from build123d import *

# Parameters (mm, degrees)
BOSS_EXTRUDE1_DEPTH     = 11
CUT_EXTRUDE1_DEPTH      = 20.874606914
CUT_EXTRUDE1_DEPTH_BACK = 20.874606914
SKETCH3_W               = 11.85
SKETCH3_H               = 1.196323822
BOSS_EXTRUDE2_DEPTH     = 11
CHAMFER1_SIZE           = 1
FILLET1_R               = 1
SKETCH4_R               = 1.175
CUT_EXTRUDE2_DEPTH      = 21.326822777
CUT_EXTRUDE3_START      = 3
SKETCH5_R               = 2.25
SKETCH5_R_2             = 1.939534676
CUT_EXTRUDE3_DEPTH      = 10
FILLET2_R               = 2
FILLET3_R               = 1
CHAMFER2_SIZE           = 1


# Some blends are built 0.0001 mm under size
with BuildPart() as part:
    # Sketch1 → Boss-Extrude1 (new body)
    with BuildSketch(Plane.XY):
        with BuildLine():
            Line((-3.15, 0), (-15, 0))
            Line((-15, 0), (-15, 7))
            Line((-15, 7), (15, 7))
            Line((15, 7), (15, 0))
            Line((15, 0), (3.15, 0))
            ThreePointArc((3.15, 0), (0, 3.15), (-3.15, 0))
        make_face()
    extrude(amount=BOSS_EXTRUDE1_DEPTH)

    # Sketch2 → Cut-Extrude1 (cut, two sides: drawn at the far end of the back side and taken through both)
    with BuildSketch(Plane.XY.offset(11).offset(-CUT_EXTRUDE1_DEPTH_BACK)):
        Polygon((-9, 5.75), (0, 7), (-15, 7), (-15, 2.504439372), align=None)
        Polygon((15, 7), (0, 7), (9, 5.75), (15, 2.504439372), align=None)
    extrude(amount=CUT_EXTRUDE1_DEPTH + CUT_EXTRUDE1_DEPTH_BACK, mode=Mode.SUBTRACT)

    # Sketch3 → Boss-Extrude2 (add)
    with BuildSketch(Plane.XY.offset(11)):
        with Locations((-9.075, -0.598161911)):
            Rectangle(SKETCH3_W, SKETCH3_H)
        with Locations((9.075, -0.598161911)):
            Rectangle(SKETCH3_W, SKETCH3_H)
    extrude(amount=-BOSS_EXTRUDE2_DEPTH)

    # Chamfer1
    chamfer1_edges = [part.edges().sort_by_distance(p)[0] for p in [
        (15, 0.654057775, 11),
        (-15, 0.654057775, 0),
        (-15, 0.654057775, 11),
        (15, 0.654057775, 0),
    ]]
    chamfer(chamfer1_edges, length=CHAMFER1_SIZE)

    # Fillet1
    fillet1_edges = [part.edges().sort_by_distance(p)[0] for p in [
        (-3.15, -1.196323822, 5.5),
        (3.15, -1.196323822, 5.5),
    ]]
    fillet(fillet1_edges, radius=FILLET1_R)

    # Sketch4 → Cut-Extrude2 (cut, through all)
    with BuildSketch(Plane.XZ.offset(1.196323822)):
        with Locations(Location((-5.25, 3.5, 0), (0, 0, 20.581969212))):
            Circle(SKETCH4_R)
        with Locations((5.25, 3.5)):
            Circle(SKETCH4_R)
        with Locations((-11, 4)):
            Circle(SKETCH4_R)
        with Locations((11, 4)):
            Circle(SKETCH4_R)
    extrude(amount=-CUT_EXTRUDE2_DEPTH, mode=Mode.SUBTRACT)

    # Sketch5 → Cut-Extrude3 (cut)
    with BuildSketch(Plane(origin=(0, 0, 0), x_dir=(1, 0, 0), z_dir=(0, 1, 0)).offset(CUT_EXTRUDE3_START)):
        with Locations(Location((-5.25, -3.5, 0), (0, 0, 180))):
            Circle(SKETCH5_R)
        with Locations((5.25, -3.5)):
            Circle(SKETCH5_R)
        with Locations(Location((-11, -4, 0), (0, 0, 27.266044451))):
            Circle(SKETCH5_R)
        with Locations((11, -4)):
            Circle(SKETCH5_R_2)
    extrude(amount=CUT_EXTRUDE3_DEPTH, mode=Mode.SUBTRACT)

    # Fillet2
    # the kernel refuses this fillet: 2 mm, written as the material it takes off along each edge
    with BuildSketch(Plane(origin=(9, 5.75, -2.170275709), x_dir=(-0.9904922731777516, 0.13756837127468827, 0), z_dir=(0, 0, 1))) as fillet2_piece_1:
        with BuildLine():
            CenterArc((FILLET2_R * 0.180856309082, FILLET2_R), FILLET2_R, 249.497020474, 20.502979526)
            Line((-FILLET2_R * 0.169399781042, FILLET2_R * 0.0633460236933), (-FILLET2_R * 0.176404902844, FILLET2_R * 0.0446129441672))
            Line((-FILLET2_R * 0.176404902844, FILLET2_R * 0.0446129441672), (-FILLET2_R * 0.00361712618164, -FILLET2_R * 0.02))
            Line((-FILLET2_R * 0.00361712618164, -FILLET2_R * 0.02), (FILLET2_R * 0.180856309082, -FILLET2_R * 0.02))
            Line((FILLET2_R * 0.180856309082, -FILLET2_R * 0.02), (FILLET2_R * 0.180856309082, 0))
        make_face()
    extrude(amount=15.340551418, mode=Mode.SUBTRACT)
    with BuildSketch(Plane(origin=(-9, 5.75, 5.139499303), x_dir=(-0.879564366325619, -0.4757799128696085, 0), z_dir=(0, 0, -1))) as fillet2_piece_2:
        with BuildLine():
            CenterArc((FILLET2_R * 0.180856309082, -FILLET2_R), FILLET2_R, 90, 20.502979526)
            Line((-FILLET2_R * 0.169399781042, -FILLET2_R * 0.0633460236933), (-FILLET2_R * 0.176404902844, -FILLET2_R * 0.0446129441672))
            Line((-FILLET2_R * 0.176404902844, -FILLET2_R * 0.0446129441672), (-FILLET2_R * 0.00361712618164, FILLET2_R * 0.02))
            Line((-FILLET2_R * 0.00361712618164, FILLET2_R * 0.02), (FILLET2_R * 0.180856309082, FILLET2_R * 0.02))
            Line((FILLET2_R * 0.180856309082, FILLET2_R * 0.02), (FILLET2_R * 0.180856309082, 0))
        make_face()
    extrude(amount=7.309775012, mode=Mode.SUBTRACT)
    with BuildSketch(Plane(origin=(-9, 5.75, 13.170275709), x_dir=(-0.879564366325619, -0.4757799128696085, 0), z_dir=(0, 0, -1))) as fillet2_piece_3:
        with BuildLine():
            CenterArc((FILLET2_R * 0.180856309082, -FILLET2_R), FILLET2_R, 90, 20.502979526)
            Line((-FILLET2_R * 0.169399781042, -FILLET2_R * 0.0633460236933), (-FILLET2_R * 0.176404902844, -FILLET2_R * 0.0446129441672))
            Line((-FILLET2_R * 0.176404902844, -FILLET2_R * 0.0446129441672), (-FILLET2_R * 0.00361712618164, FILLET2_R * 0.02))
            Line((-FILLET2_R * 0.00361712618164, FILLET2_R * 0.02), (FILLET2_R * 0.180856309082, FILLET2_R * 0.02))
            Line((FILLET2_R * 0.180856309082, FILLET2_R * 0.02), (FILLET2_R * 0.180856309082, 0))
        make_face()
    extrude(amount=10.309775012, mode=Mode.SUBTRACT)
    with BuildSketch(Plane(origin=(0, 7, 12.666666667), x_dir=(-0.9904922731777517, -0.13756837127468774, 0), z_dir=(0, 0, -1))) as fillet2_piece_4:
        with BuildLine():
            CenterArc((FILLET2_R * 0.138888888889, -FILLET2_R), FILLET2_R, 90, 15.814325406)
            Line((-FILLET2_R * 0.133631928674, -FILLET2_R * 0.0378501135503), (-FILLET2_R * 0.139082345025, -FILLET2_R * 0.0186071158213))
            Line((-FILLET2_R * 0.139082345025, -FILLET2_R * 0.0186071158213), (-FILLET2_R * 0.00277777777778, FILLET2_R * 0.02))
            Line((-FILLET2_R * 0.00277777777778, FILLET2_R * 0.02), (FILLET2_R * 0.138888888889, FILLET2_R * 0.02))
            Line((FILLET2_R * 0.138888888889, FILLET2_R * 0.02), (FILLET2_R * 0.138888888889, 0))
        make_face()
    extrude(amount=14.333333333, mode=Mode.SUBTRACT)
    with BuildSketch(Plane(origin=(-15, 2.504439372, -6.151996245), x_dir=(0.8795643663256194, 0.4757799128696078, 0), z_dir=(0, 0, 1))) as fillet2_piece_5:
        with BuildLine():
            CenterArc((FILLET2_R * 0.595999687118, -FILLET2_R), FILLET2_R, 90, 61.589857771)
            Line((-FILLET2_R * 0.283564679207, -FILLET2_R * 0.52422008713), (-FILLET2_R * 0.301155966534, -FILLET2_R * 0.514704488873))
            Line((-FILLET2_R * 0.301155966534, -FILLET2_R * 0.514704488873), (-FILLET2_R * 0.0119199937424, FILLET2_R * 0.02))
            Line((-FILLET2_R * 0.0119199937424, FILLET2_R * 0.02), (FILLET2_R * 0.595999687118, FILLET2_R * 0.02))
            Line((FILLET2_R * 0.595999687118, FILLET2_R * 0.02), (FILLET2_R * 0.595999687118, 0))
        make_face()
    extrude(amount=23.303992491, mode=Mode.SUBTRACT)
    with BuildSketch(Plane(origin=(15, 2.504439372, -6.151996245), x_dir=(-0.87956436632562, 0.47577991286960686, 0), z_dir=(0, 0, 1))) as fillet2_piece_6:
        with BuildLine():
            CenterArc((FILLET2_R * 0.595999687118, FILLET2_R), FILLET2_R, 208.410142229, 61.589857771)
            Line((-FILLET2_R * 0.283564679207, FILLET2_R * 0.52422008713), (-FILLET2_R * 0.301155966534, FILLET2_R * 0.514704488873))
            Line((-FILLET2_R * 0.301155966534, FILLET2_R * 0.514704488873), (-FILLET2_R * 0.0119199937424, -FILLET2_R * 0.02))
            Line((-FILLET2_R * 0.0119199937424, -FILLET2_R * 0.02), (FILLET2_R * 0.595999687118, -FILLET2_R * 0.02))
            Line((FILLET2_R * 0.595999687118, -FILLET2_R * 0.02), (FILLET2_R * 0.595999687118, 0))
        make_face()
    extrude(amount=23.303992491, mode=Mode.SUBTRACT)

    # Fillet3
    fillet3_edges = [part.edges().sort_by_distance(p)[0] for p in [
        (15, -1.196323822, 5.5),
        (-15, -1.196323822, 5.5),
    ]]
    fillet(fillet3_edges, radius=FILLET3_R)

    # Chamfer2
    chamfer2_edges = [part.edges().sort_by_distance(p)[0] for p in [
        (-11.634854678, 4.324736566, 0),
        (-11.634854678, 4.324736566, 11),
        (-8.989888283, 5.719170071, 0),
        (-8.989888283, 5.719170071, 11),
        (-4.458431595, 6.38077339, 0),
        (-4.458431595, 6.38077339, 11),
        (11.634854678, 4.324736566, 11),
        (11.634854678, 4.324736566, 0),
        (0, 6.980802017, 0),
        (0, 6.980802017, 11),
        (8.989888283, 5.719170071, 0),
        (8.989888283, 5.719170071, 11),
        (4.458431595, 6.38077339, 11),
        (4.458431595, 6.38077339, 0),
        (-9.075, -1.196323822, 0),
        (9.075, -1.196323822, 0),
        (-3.442893219, -0.903430603, 0),
        (-3.442893219, -0.903430603, 11),
        (3.442893219, -0.903430603, 11),
        (3.442893219, -0.903430603, 0),
        (-3.15, -0.098161911, 0),
        (3.15, -0.098161911, 0),
        (0, 3.15, 0),
        (0, 3.15, 11),
        (-9.075, -1.196323822, 11),
        (9.075, -1.196323822, 11),
        (-3.15, -0.098161911, 11),
        (3.15, -0.098161911, 11),
        (-13.975873835, 3.058197787, 0),
        (-13.975873835, 3.058197787, 11),
        (13.975873835, 3.058197787, 0),
        (13.975873835, 3.058197787, 11),
    ]]
    chamfer(chamfer2_edges, length=CHAMFER2_SIZE - 0.0001)  # a hair under: the kernel refuses the full size


solid = part.part
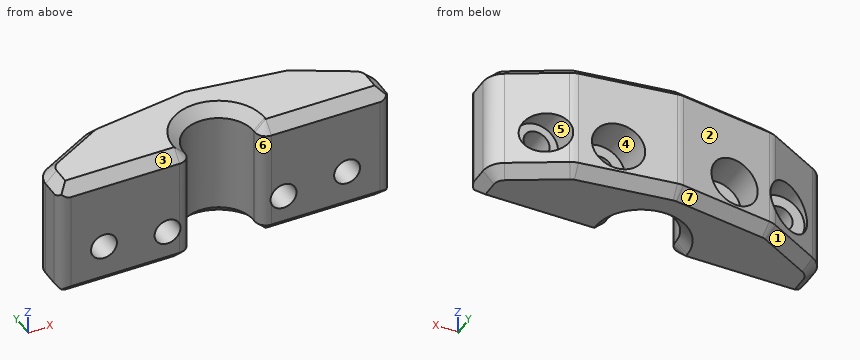
For this review, take the finished solid that the model builds, in its own axes (mm). Face numbers are marked on the shaded views. A direction names the side the tool comes from. Round coordinates to 2 decimals unless told otherwise and drop trailing zeros. Write each loop counter-clockwise with the first axis right and the second up, starting at its lowest first coordinate (ties: lowest second). Pieces come first, ordered by that corner, then holes. Notation, with made-up numbers: (52, 54.25) -> (103, 54.25) arc R30 cw to (103, 85.25) -> close; hole circle Ø2 at (23.25, 4.5). An arc over 180 degrees is marked (long way). Use CSV: the item, a comma, the result in double quotes.
(1) Draft analysis for pull direction Z (two halves, no side actions). For the marked faces 1, 2, 3 and 4, state which applies: +Z half, -Z half, draft (parallel to the pull), parting line (faces both ways), or undercut.
Computed values:
face 1,"-Z half"
face 2,"draft"
face 3,"+Z half"
face 4,"undercut"
(2) Consider section D-D, the plane x = 8. Give the boundary of the cut face in (y, z).
Computed values:
outline,"(-1.2, 1) -> (-0.2, 0) -> (4.88, 0) -> (5.89, 1) -> (5.89, 10) -> (4.88, 11) -> (-0.2, 11) -> (-1.2, 10) -> close"
(3) For the marked faces 5, 6 and 7, list the 3-axis set-ups (+Z, -Z, +X, -X, +Y, -Y) from which the entire face can be reached by the end or side of a thin tool; tool diameter is ignored.
Computed values:
face 5,"+Y"
face 6,"+Z, -Z, -Y"
face 7,"-Z, -X, +Y"
(4) Consider section A-A, the plane z = 9.25. Give the boundary of the cut face in (x, y).
Computed values:
outline,"(-15, -0.2) arc R1 ccw to (-14, -1.2) -> (-4.15, -1.2) arc R1 ccw to (-3.15, -0.2) -> (-3.15, 0) arc R3.15 cw to (3.15, 0) -> (3.15, -0.2) arc R1 ccw to (4.15, -1.2) -> (14, -1.2) arc R1 ccw to (15, -0.2) -> (15, 1.31) arc R2 ccw to (13.95, 3.07) -> (9.32, 5.58) arc R2 ccw to (8.64, 5.8) -> (0.28, 6.96) arc R2 ccw to (-0.28, 6.96) -> (-8.64, 5.8) arc R2 ccw to (-9.32, 5.58) -> (-13.95, 3.07) arc R2 ccw to (-15, 1.31) -> close"
(5) Consider section B-B, the plane x = -11. Give the boundary of the cut face in (y, z) (3 decimals), plus the area to 3 significant figures.
Computed values:
outline,"(-1.196, 1) -> (-0.196, 0) -> (3.531, 0) -> (4.668, 1) -> (4.668, 1.75) -> (3, 1.75) -> (3, 2.825) -> (-1.196, 2.825) -> close; (-1.196, 5.175) -> (3, 5.175) -> (3, 6.25) -> (4.668, 6.25) -> (4.668, 10) -> (3.531, 11) -> (-0.196, 11) -> (-1.196, 10) -> close"
area,"45.0 mm²"
(6) Consider section C-C, the plane y = -0.5. Give the number of separate pieces and of enclosed holes in the cut face, plus the area to 3 significant figures.
Computed values:
separate pieces,"2"
enclosed holes,"4"
area,"225 mm²"
(7) To check wall thickness, follow L1, parallel to Z at x = 5.25, y = 5.05; L2, parallel to Z at x = -11, y = 0.75 (3 decimals); L3, parallel to X at y = 1.25, z = 3.5 (3 decimals). State the ranges of each line that lie inside material, in increasing order. Write a range as [from, to].
Computed values:
L1,"[0, 1.25], [5.75, 11]"
L2,"[0, 2.825], [5.175, 11]"
L3,"[-15, -12.063], [-9.937, -6.425], [-4.075, -2.891], [2.891, 4.075], [6.425, 9.937], [12.063, 15]"
(8) Clearance check with flat-ended pins moving along their axes: P1, Ø6, axis at x = -10, z = 4, coming from the +Y side; P2, Ø4, axis at x = -11, z = 4, coming from the -Y side; P3, Ø1, axis at y = 2, z = 7.5, coming from the -X side; P4, Ø2.5, axis at x = 11, z = 4, coming from the +Y side. State where each tip first meets the part, or that it passes through.
Computed values:
P1,"y = 6.01"
P2,"y = -1.2"
P3,"x = -14.99"
P4,"y = 3"
